Read the model definition and answer for the solid it produces. Units are mm, in the model's axes. A direction names the side the tool comes from. Give positions to 0.01 mm unless a question says otherwise; leave off trailing zeros. Loops run counter-clockwise (first coordinate to the right, second up) from the corner with the lowest first, then second, coordinate; pieces in that order, holes last.
(1) Determine the mould class of faces 6 (the face through (-8, -64, 1.709)), 7 (the face through (-16.81, 35.25, 0.87)), 8 (the face through (4.66, -23.18, 0.84)) for opening direction X: pulls with the +X half, pulls with the -X half, needs draft (parallel to the pull), parting line crosses it, or undercut.
(2) Which of the six approach directions +Z, -Z, +X, -X, +Y, -Y give full straight-line access (tool end or side, diameter ignored) to faces 1 (the face through (-20, -20.32, -1)), 2 (the face through (20, -20.32, -1)), 3 (the face through (-5.11, -23.18, 0.84)), 4 (the face through (-8, -64, 0)), 5 (the face through (-0.3, -166.997, 0.5))?
(3) Each of these flat-tipped pins is pushed along its axis until it touches: P1, Ø3.5, axis at x = -10.83, y = -155.88, coming from the +Z side; P2, Ø10, axis at x = 15.5, y = -30, coming from the -Z side; P3, Ø10.5, axis at x = 6, y = -17, coming from the -Z side; P4, Ø1.9, axis at y = -21.5, z = 1.5, coming from the -X side. Where does it stop, or does it pass through?
(4) Find section A-A, the plane y = -65.5. Write down the section's boundary in (x, z), then the cut area to 3 significant figures.
(5) Straight lines are drawn through the part: probe 1 along Y at (x, z) = (5, 0.15); probe 2 along Y at (x, z) = (-0.5, 0.5); probe 3 along Y at (x, z) = (-11, 0.2). For each, find the intervals that lie inside material, in ascending order.
(6) Find section B-B, the plane y = -7. Write down the section's boundary in (x, z), then the cut area to 3 significant figures.
```python
from build123d import *

# Parameters (mm, degrees)
F0_W     = 35.433
F0_H     = 203.2
F0_R     = 1.8288
F0_R_2   = 1.35255
F0_W_2   = 15.305659
F0_H_2   = 130.1990486724
F0_R_3   = 1.7272
F0_W_3   = 19.558
F0_H_3   = 40.64
F1_DEPTH = 1.70942
F3_DEPTH = 146.6772986724
F4_R     = 3.175
F5_W     = 6.35
F5_H     = 6.35
F6_DEPTH = 1.70942


with BuildPart() as f1:
    # F0 (on Top) → F1 (new body)
    with BuildSketch(Plane.XY):
        with Locations((0, -65.3972986724)):
            Rectangle(F0_W, F0_H)
        with Locations((-14.5415, -163.8222986724)):
            Circle(F0_R, mode=Mode.SUBTRACT)
        with Locations((-10.8278295, -155.8847986724)):
            Circle(F0_R_2, mode=Mode.SUBTRACT)
        with Locations((14.5415, -163.8222986724)):
            Circle(F0_R, mode=Mode.SUBTRACT)
        with Locations((0, -93.9602743362)):
            Rectangle(F0_W_2, F0_H_2, mode=Mode.SUBTRACT)
        with Locations((-4.8895, -24.892)):
            Circle(F0_R_3, mode=Mode.SUBTRACT)
        with Locations((-14.5415, -11.7291104)):
            Circle(F0_R, mode=Mode.SUBTRACT)
        with Locations((-14.5415, 33.0277013276)):
            Circle(F0_R_2, mode=Mode.SUBTRACT)
        with Locations((-4.8895, 24.892)):
            Circle(F0_R_3, mode=Mode.SUBTRACT)
        with Locations((4.8895, -24.892)):
            Circle(F0_R_3, mode=Mode.SUBTRACT)
        Rectangle(F0_W_3, F0_H_3, mode=Mode.SUBTRACT)
        with Locations((4.8895, 24.892)):
            Circle(F0_R_3, mode=Mode.SUBTRACT)
        with Locations((14.5415, -11.7291104)):
            Circle(F0_R, mode=Mode.SUBTRACT)
        with Locations((14.5415, 33.0277013276)):
            Circle(F0_R_2, mode=Mode.SUBTRACT)
    extrude(amount=F1_DEPTH)

    # F2 (on face) → F3 (join, through all)
    with BuildSketch(Plane.XZ.offset(166.9972986724)):
        with BuildLine():
            ThreePointArc((-19.1192160061, -0.5810239939), (-18.4756444321, -0.1510032162), (-17.7165, 0))
            Line((-17.7165, 0), (-17.7165, 1.70942))
            ThreePointArc((-17.7165, 1.70942), (-19.1298111451, 1.4282949343), (-20.32795848, 0.62771848))
            Line((-20.32795848, 0.62771848), (-22.5730225103, -1.6173455503))
            Line((-22.5730225103, -1.6173455503), (-21.3642800364, -2.8260880242))
            Line((-21.3642800364, -2.8260880242), (-19.1192160061, -0.5810239939))
        make_face()
        with BuildLine():
            Line((17.7165, 1.70942), (17.7165, 0))
            ThreePointArc((17.7165, 0), (18.4756444321, -0.1510032162), (19.1192160061, -0.5810239939))
            Line((19.1192160061, -0.5810239939), (21.3642800364, -2.8260880242))
            Line((21.3642800364, -2.8260880242), (22.5730225103, -1.6173455503))
            Line((22.5730225103, -1.6173455503), (20.32795848, 0.62771848))
            ThreePointArc((20.32795848, 0.62771848), (19.1298111451, 1.4282949343), (17.7165, 1.70942))
        make_face()
    extrude(amount=-F3_DEPTH)

    # F4
    f4_edges = [f1.edges().sort_by_distance(p)[0] for p in [
        (17.7165, 36.202701, 0.85471),
        (-17.7165, 36.202701, 0.85471),
    ]]
    fillet(f4_edges, radius=F4_R)

    # F5 (on face) → F6 (cut, through all)
    with BuildSketch(Plane.XY.offset(1.70942)):
        with Locations((0, 33.0277013276)):
            Rectangle(F5_W, F5_H)
        with BuildLine():
            Line((1.016, -23.749), (1.016, -20.32))
            Line((1.016, -20.32), (-1.016, -20.32))
            Line((-1.016, -20.32), (-1.016, -23.749))
            ThreePointArc((-1.016, -23.749), (0, -24.765), (1.016, -23.749))
        make_face()
        with BuildLine():
            Line((-1.016, 20.32), (1.016, 20.32))
            Line((1.016, 20.32), (1.016, 23.749))
            ThreePointArc((1.016, 23.749), (0, 24.765), (-1.016, 23.749))
            Line((-1.016, 23.749), (-1.016, 20.32))
        make_face()
    extrude(amount=-F6_DEPTH, mode=Mode.SUBTRACT)


solid = f1.part
```
Entries:
1. face 6: needs draft
1. face 7: pulls with the -X half
1. face 8: undercut
2. face 1: +Z, -Z, -X, +Y
2. face 2: +Z, -Z, +X, +Y
2. face 3: +Z, -Z
2. face 4: -Z, +Y, -Y
2. face 5: +Z, -Z, +X, -X, -Y
3. P1: stops at z = 1.71
3. P2: stops at z = -1.96
3. P3: stops at z = 0
3. P4: stops at x = -20.41
4. outline: (-22.57, -1.62) - (-21.36, -2.83) - (-19.12, -0.58) arc R1.98 cw to (-17.72, 0) - (-7.65, 0) - (-7.65, 1.71) - (-17.72, 1.71) arc R3.69 ccw to (-20.33, 0.63) - close; (7.65, 0) - (17.72, 0) arc R1.98 cw to (19.12, -0.58) - (21.36, -2.83) - (22.57, -1.62) - (20.33, 0.63) arc R3.69 ccw to (17.72, 1.71) - (7.65, 1.71) - close
4. area: 52.9 mm2
5. probe 1: y = -167 to -159.06, -28.86 to -26.62, -23.17 to -20.32, 20.32 to 23.17, 26.62 to 36.2
5. probe 2: y = -167 to -159.06, -28.86 to -24.63, 24.63 to 29.85
5. probe 3: y = -167 to -157.23, -154.54 to 36.2
6. outline: (-17.72, 0) - (-9.78, 0) - (-9.78, 1.71) - (-17.72, 1.71) - close; (9.78, 0) - (17.72, 0) - (17.72, 1.71) - (9.78, 1.71) - close
6. area: 27.1 mm2
